Part model, mm, in its own coordinate system. Face numbers are marked on the shaded views. A direction names the side the tool comes from. Coordinates: 2 decimals unless noted, no trailing zeros. Order: outer loops, then holes, each group sorted by start corner. A loop starts at its lowest first (then second) coordinate and runs counter-clockwise, first axis right, second up.
1) Mould opens along X. For the marked faces 1, 2, 3 and 4 say: +X half, -X half, draft (parallel to the pull), parting line (faces both ways), or undercut.
2) Wall check: L1, parallel to Y at x = 18.75, z = 0; L2, parallel to Z at x = 9, y = 64.5; L3, parallel to X at y = 92, z = 11.5. Give the ranges that are in metal, low to high.
3) Pin check, flat tips, straight feed: pin 1 Ø10 at (x, y) = (-14.5, 74) entering from +Z; pin 2 Ø6 at (x, y) = (-18, 79.5) entering from +Z; pin 3 Ø6 at (y, z) = (76, 10) entering from -X; pin 4 Ø3.5 at (y, z) = (35, 0) entering from +X (3 decimals). Stop position of each tip, or through.
4) Cut at B-B (z = 0). List the corners of the cut face in (x, y).
5) Cut at D-D (z = 14). List the corners of the cut face in (x, y), and give its area (3 significant figures).
6) Cut at A-A (x = 0). List the corners of the cut face in (y, z), and give its area (3 significant figures).
7) Cut at C-C (y = 79). List the corners of the cut face in (x, z), and give its area (3 significant figures).
8) Tool access for the marked faces 5 and 6: list every direction of +Z, -Z, +X, -X, +Y, -Y with a clear straight run to the whole face (end or side of a thin tool).
```python
from build123d import *

# Parameters (mm, degrees)
SKETCH1_R               = 23.9
SKETCH1_R_2             = 18.9
BOSS_EXTRUDE1_DEPTH     = 100
SKETCH2_R               = 2.3
CUT_EXTRUDE1_DEPTH      = 24.9
CUT_EXTRUDE1_DEPTH_BACK = 24.9
FILLET1_R               = 2


with BuildPart() as part:
    # Sketch1 → Boss-Extrude1 (new body)
    with BuildSketch(Plane(origin=(0, 0, 0), x_dir=(1, 0, 0), z_dir=(0, 1, 0))):
        Circle(SKETCH1_R)
        Circle(SKETCH1_R_2, mode=Mode.SUBTRACT)
        with BuildLine():
            Line((-15, -11.498260738), (-15, 11.498260738))
            ThreePointArc((-15, 11.498260738), (-18.9, 0), (-15, -11.498260738))
        make_face()
        with BuildLine():
            ThreePointArc((18.9, 0), (17.898463621, 6.070831903), (15, 11.498260738))
            Line((15, 11.498260738), (15, -11.498260738))
            ThreePointArc((15, -11.498260738), (17.898463621, -6.070831903), (18.9, 0))
        make_face()
    extrude(amount=BOSS_EXTRUDE1_DEPTH)

    # Sketch2 → Cut-Extrude1 (cut, two sides)
    with BuildSketch(Plane(origin=(0, 0, 0), x_dir=(0, 0, -1), z_dir=(1, 0, 0))) as cut_extrude1_sk:
        with Locations((0, 15)):
            Circle(SKETCH2_R)
        with Locations((0, 35)):
            Circle(SKETCH2_R)
    extrude(amount=CUT_EXTRUDE1_DEPTH, mode=Mode.SUBTRACT)
    extrude(cut_extrude1_sk.sketch, amount=-CUT_EXTRUDE1_DEPTH_BACK, mode=Mode.SUBTRACT)

    # Fillet1
    fillet1_edges = [part.edges().sort_by_distance(p)[0] for p in [
        (15, 50, 11.498260738),
        (15, 50, -11.498260738),
        (-15, 50, -11.498260738),
        (-15, 50, 11.498260738),
    ]]
    fillet(fillet1_edges, radius=FILLET1_R)


solid = part.part
```
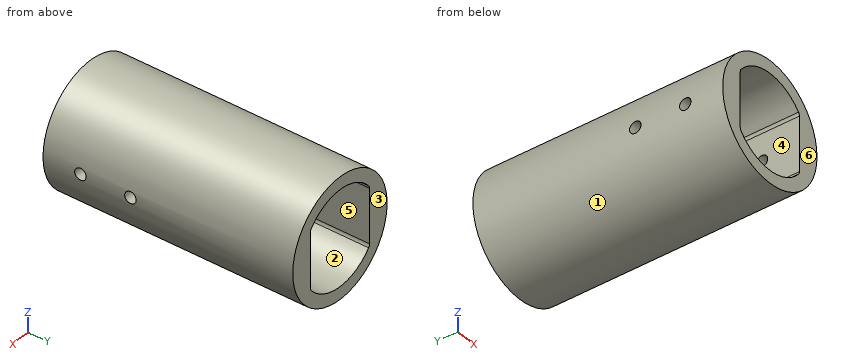
Geometry check:
1. face 1: parting line
1. face 2: undercut
1. face 3: draft
1. face 4: undercut
2. L1: y = 0 to 12.7, 17.3 to 32.7, 37.3 to 100
2. L2: z = -22.14 to -16.62, 16.62 to 22.14
2. L3: x = -20.95 to -14.87, 14.87 to 20.95
3. pin 1: stops at z = 21.93
3. pin 2: stops at z = 18.61
3. pin 3: stops at x = -22.85
3. pin 4: passes through
4. outline: (-23.9, 0) - (-15, 0) - (-15, 12.7) - (-23.9, 12.7) - close; (-23.9, 17.3) - (-15, 17.3) - (-15, 32.7) - (-23.9, 32.7) - close; (-23.9, 37.3) - (-15, 37.3) - (-15, 100) - (-23.9, 100) - close; (15, 0) - (23.9, 0) - (23.9, 12.7) - (15, 12.7) - close; (15, 17.3) - (23.9, 17.3) - (23.9, 32.7) - (15, 32.7) - close; (15, 37.3) - (23.9, 37.3) - (23.9, 100) - (15, 100) - close
5. outline: (-19.37, 0) - (-12.7, 0) - (-12.7, 100) - (-19.37, 100) - close; (12.7, 0) - (19.37, 0) - (19.37, 100) - (12.7, 100) - close
5. area: 1,330 mm2
6. outline: (0, -23.9) - (100, -23.9) - (100, -18.9) - (0, -18.9) - close; (0, 18.9) - (100, 18.9) - (100, 23.9) - (0, 23.9) - close
6. area: 1,000 mm2
7. outline: circle Ø47.8 at (0, 0); hole (-15, -10.8) arc R2 ccw to (-14.54, -12.08) arc R18.9 ccw to (14.54, -12.08) arc R2 ccw to (15, -10.8) - (15, 10.8) arc R2 ccw to (14.54, 12.08) arc R18.9 ccw to (-14.54, 12.08) arc R2 ccw to (-15, 10.8) - close
7. area: 795 mm2
8. face 5: +Y, -Y
8. face 6: +Z, -Z, +X, -X, -Y
